For this review, take the finished solid that the model builds, in its own axes (mm). A direction names the side the tool comes from. Give positions to 0.01 mm unless a question says otherwise; leave off trailing zeros. Loops run counter-clockwise (first coordinate to the right, second up) from the corner with the lowest first, then second, coordinate; pieces in that order, holes last. Notation, with made-up numbers: (-37, -15.75) - (-31, -15.75) arc R10 ccw to (-31, -4.75) - close; hole circle Ø6 at (-10.75, 3.5). An arc over 180 degrees is marked (long way). Answer in a Markdown table with one row per item.
```python
from build123d import *

# Parameters (mm, degrees)
F2_DEPTH = 15


with BuildPart() as f2:
    # F1 (on Top) → F2 (new body)
    with BuildSketch(Plane.XY):
        Polygon((-39.3307432532, 0), (-24.3307432532, 0), (-24.3307432532, 5), (-24.3307432532, 6), (-25.3307432532, 6), (-25.3307432532, 1), (-38.3307432532, 1), (-38.3307432532, 14), (-25.3307432532, 14), (-24.3307432532, 14), (-24.3307432532, 15), (-39.3307432532, 15), align=None)
        Polygon((-24.3307432532, 6), (-24.3307432532, 5), (-9.3307432532, 5), (-9.3307432532, 6), (-10.3307432532, 6), (-23.3307432532, 6), align=None)
        Polygon((-9.3307432532, 6), (-9.3307432532, 5), (-9.3307432532, 0), (5.6692567468, 0), (5.6692567468, 15), (-9.3307432532, 15), (-9.3307432532, 14), (-8.3307432532, 14), (4.6692567468, 14), (4.6692567468, 1), (-8.3307432532, 1), (-8.3307432532, 6), align=None)
        Polygon((-24.3307432532, 20), (-24.3307432532, 15), (-24.3307432532, 14), (-23.3307432532, 14), (-23.3307432532, 19), (-10.3307432532, 19), (-10.3307432532, 14), (-9.3307432532, 14), (-9.3307432532, 15), (-9.3307432532, 20), align=None)
    extrude(amount=F2_DEPTH)


solid = f2.part
```
1. Mouldability with a two-part tool opening along X and no side actions: class faces 1 (the face through (-9.331, 3, 7)), 2 (the face through (-18.6, 5.6, 0)), 3 (the face through (-24.331, 18, 7)) as released by +X, released by -X, zero draft, split by the parting line, or undercut.
Values:
| item | result |
|---|---|
| face 1 | undercut |
| face 2 | zero draft |
| face 3 | released by -X |
2. For faces 4 (the face through (-32, 15, 7)), 5 (the face through (-17, 5, 7)), 6 (the face through (5.669, 7, 7)), 7 (the face through (-8.331, 3, 7)), 8 (the face through (-2, 15, 7)), list the 3-axis set-ups (+Z, -Z, +X, -X, +Y, -Y) from which the entire face can be reached by the end or side of a thin tool; tool diameter is ignored.
Values:
| item | result |
|---|---|
| face 4 | +Z, -Z, -X, +Y |
| face 5 | +Z, -Z, -Y |
| face 6 | +Z, -Z, +X, +Y, -Y |
| face 7 | +Z, -Z |
| face 8 | +Z, -Z, +X, +Y |
3. We need section C-C, the plane x = -1. Give the boundary of the cut face in (y, z).
Values:
| item | result |
|---|---|
| outline | (0, 0) - (1, 0) - (1, 15) - (0, 15) - close; (14, 0) - (15, 0) - (15, 15) - (14, 15) - close |
4. We need section D-D, the plane y = 10.5. Give the boundary of the cut face in (x, z), and give its area (3 significant figures).
Values:
| item | result |
|---|---|
| outline | (-39.33, 0) - (-38.33, 0) - (-38.33, 15) - (-39.33, 15) - close; (4.67, 0) - (5.67, 0) - (5.67, 15) - (4.67, 15) - close |
| area | 30.0 mm^2 |
5. We need section A-A, the plane y = 4.5. Give the boundary of the cut face in (x, z).
Values:
| item | result |
|---|---|
| outline | (-39.33, 0) - (-38.33, 0) - (-38.33, 15) - (-39.33, 15) - close; (-25.33, 0) - (-24.33, 0) - (-24.33, 15) - (-25.33, 15) - close; (-9.33, 0) - (-8.33, 0) - (-8.33, 15) - (-9.33, 15) - close; (4.67, 0) - (5.67, 0) - (5.67, 15) - (4.67, 15) - close |
6. We need section B-B, the plane z = 9.5. Give the boundary of the cut face in (x, y), and give its area (3 significant figures).
Values:
| item | result |
|---|---|
| outline | (-39.33, 0) - (-24.33, 0) - (-24.33, 5) - (-9.33, 5) - (-9.33, 0) - (5.67, 0) - (5.67, 15) - (-9.33, 15) - (-9.33, 20) - (-24.33, 20) - (-24.33, 15) - (-39.33, 15) - close; hole (-38.33, 1) - (-25.33, 1) - (-25.33, 6) - (-8.33, 6) - (-8.33, 1) - (4.67, 1) - (4.67, 14) - (-10.33, 14) - (-10.33, 19) - (-23.33, 19) - (-23.33, 14) - (-38.33, 14) - close |
| area | 136 mm^2 |
7. Wall thickness on line 1 (X direction, y = 3.25, z = 4.75); line 2 (Y direction, x = -16, z = 1); line 3 (X direction, y = 18, z = 14): over which ranges is each line inside the solid? List them lowest first. Write a range as [from, to].
Values:
| item | result |
|---|---|
| line 1 | x = [-39.33, -38.33], [-25.33, -24.33], [-9.33, -8.33], [4.67, 5.67] |
| line 2 | y = [5, 6], [19, 20] |
| line 3 | x = [-24.33, -23.33], [-10.33, -9.33] |
8. Clearance check with flat-ended pins moving along their axes: pin 1 (5 mm diameter, centred on x = -32.5, y = 9.5, fed in from +Z); pin 2 (2.5 mm diameter, centred on y = 16.5, z = 5, fed in from +X); pin 3 (7.5 mm diameter, centred on x = -3.5, z = 9, fed in from +Y); pin 4 (7.5 mm diameter, centred on x = -14.5, z = 4, fed in from -Y). State where each tip first meets the part, or that it passes through.
Values:
| item | result |
|---|---|
| pin 1 | passes through |
| pin 2 | stops at x = -9.33 |
| pin 3 | stops at y = 15 |
| pin 4 | stops at y = 5 |
